Read the model definition and answer for the solid it produces. Units are mm, in the model's axes. Face numbers are marked on the shaded views. A direction names the side the tool comes from. Round coordinates to 2 decimals unless told otherwise and drop trailing zeros. Write each loop counter-clockwise with the first axis right and the second up, starting at its lowest first coordinate (ties: lowest second). Pieces come first, ordered by that corner, then holes. Notation, with made-up numbers: (59.25, 63) - (79.25, 63) arc R17 ccw to (79.25, 93) - close; hole circle Ø4 at (67.25, 75). An arc over 180 degrees is marked (long way). One line per item, written item: value. Start each with the question number.
(1) A cutting plane is placed at A-A, the plane z = 2. Determine the outline of the cut face in (x, y).
(2) A cutting plane is placed at B-B, the plane y = 41.75. Determine the outline of the cut face in (x, z), plus the area to 3 significant figures.
(3) Flat-ended cylindrical pins translate along their axes: pin 1 Ø4 at (y, z) = (43.5, 3) entering from +X; pin 2 Ø5 at (x, y) = (-19.5, 31) entering from -Z; pin 3 Ø2 at (x, z) = (48.5, 2) entering from +Y; pin 4 Ø5 at (y, z) = (-25, -37.41) entering from +X. Find the tip coordinate at first contact, or state that the pin passes through.
(4) A cutting plane is placed at C-C, the plane z = -37.41. Determine the outline of the cut face in (x, y) (3 decimals), plus the area to 3 significant figures.
(5) For the marked faces 1, 2 and 3, determine the directions among +Z, -Z, +X, -X, +Y, -Y from which every point of the face is accessible in a straight line to the end or side of a thin tool.
(6) Find the intervals of material crossed by L1, parallel to Y at x = 0, z = -37.41; L2, parallel to Y at x = 30.5, z = 2; L3, parallel to X at y = -32, z = -43.5 (3 decimals), in increasing order.
(7) A cutting plane is placed at D-D, the plane x = 29.5. Determine the outline of the cut face in (y, z).
from build123d import *

# Parameters (mm, degrees)
SKETCH1_W           = 100
SKETCH1_H           = 75
BOSS_EXTRUDE1_DEPTH = 4
SKETCH2_R           = 2
BOSS_EXTRUDE2_DEPTH = 30
SKETCH3_W           = 50
SKETCH3_H           = 25
BOSS_EXTRUDE3_DEPTH = 6.665
CUT_EXTRUDE2_START  = -13.33
CUT_EXTRUDE2_DEPTH  = 13.33
SKETCH5_R           = 4.2
CUT_EXTRUDE3_DEPTH  = 89.340164846


# Read off the part's stored shape, not the designer's step: Cut-Extrude2
with BuildPart() as part:
    # Sketch1 → Boss-Extrude1 (new body)
    with BuildSketch(Plane.XY):
        Rectangle(SKETCH1_W, SKETCH1_H)
    extrude(amount=BOSS_EXTRUDE1_DEPTH)

    # Sketch2 → Boss-Extrude2 (add)
    with BuildSketch(Plane(origin=(45, 0, 0), x_dir=(0, 0, -1), z_dir=(1, 0, 0))):
        with BuildLine():
            Line((-4, 38.285898385), (-4, 37.428468659))
            Line((-4, 37.428468659), (0, 37.428468659))
            Line((0, 37.428468659), (0, 38.285898385))
            ThreePointArc((0, 38.285898385), (-2, 45.75), (-4, 38.285898385))
        make_face()
        with Locations((-2, 41.75)):
            Circle(SKETCH2_R, mode=Mode.SUBTRACT)
    boss_extrude2 = extrude(amount=-BOSS_EXTRUDE2_DEPTH)

    # Mirror1: Boss-Extrude2 across plane
    add(boss_extrude2.mirror(Plane.ZY))

    # Sketch3 → Boss-Extrude3 (add, symmetric)
    with BuildSketch(Plane.ZY):
        with Locations((-25, -25)):
            Rectangle(SKETCH3_W, SKETCH3_H)
    extrude(amount=BOSS_EXTRUDE3_DEPTH, both=True)

    # Cut-Extrude2 outline → Cut-Extrude2 (cut)
    with BuildSketch(Plane.ZY.offset(6.665).offset(CUT_EXTRUDE2_START)):
        with BuildLine():
            Line((-50, -37.5), (-38.919370818, -37.5))
            ThreePointArc((-38.919370818, -37.5), (-46.831015832, -33.352603885), (-50, -25.000804036))
            Line((-50, -25.000804036), (-50, -37.5))
        make_face()
        with BuildLine():
            Line((-50, -12.5), (-50, -25.000804036))
            ThreePointArc((-50, -25.000804036), (-46.826545708, -16.643964506), (-38.905994132, -12.5))
            Line((-38.905994132, -12.5), (-50, -12.5))
        make_face()
    extrude(amount=CUT_EXTRUDE2_DEPTH, mode=Mode.SUBTRACT)

    # Sketch5 → Cut-Extrude3 (cut, through all)
    with BuildSketch(Plane.ZY.offset(6.665)):
        with Locations((-37.41, -25.000804036)):
            Circle(SKETCH5_R)
    extrude(amount=-CUT_EXTRUDE3_DEPTH, mode=Mode.SUBTRACT)


solid = part.part
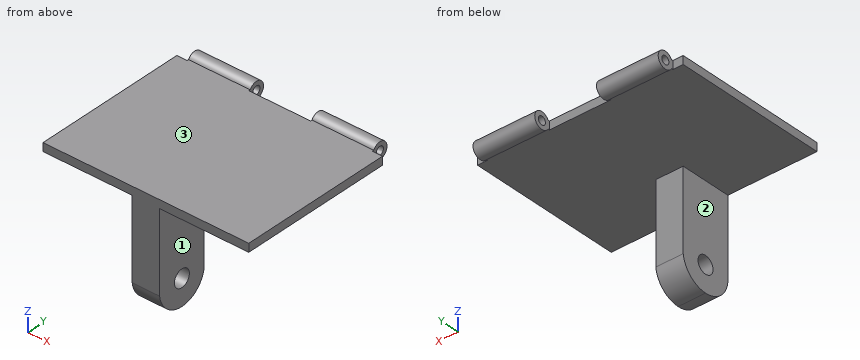
Here are the results:
1. outline: (-50, -37.5) - (50, -37.5) - (50, 37.5) - (45, 37.5) - (45, 39.75) - (15, 39.75) - (15, 37.5) - (-15, 37.5) - (-15, 39.75) - (-45, 39.75) - (-45, 37.5) - (-50, 37.5) - close; (-45, 43.75) - (-15, 43.75) - (-15, 45.75) - (-45, 45.75) - close; (15, 43.75) - (45, 43.75) - (45, 45.75) - (15, 45.75) - close
2. outline: (-45, -2) - (-15, -2) - (-15, 0) - (-45, 0) - close; (-45, 4) - (-15, 4) - (-15, 6) - (-45, 6) - close; (15, -2) - (45, -2) - (45, 0) - (15, 0) - close; (15, 4) - (45, 4) - (45, 6) - (15, 6) - close
2. area: 240 mm²
3. pin 1: x = 45
3. pin 2: z = 0
3. pin 3: y = 37.5
3. pin 4: through
4. outline: (-6.665, -37.5) - (6.665, -37.5) - (6.665, -29.201) - (-6.665, -29.201) - close; (-6.665, -20.801) - (6.665, -20.801) - (6.665, -12.5) - (-6.665, -12.5) - close
4. area: 221 mm²
5. face 1: -Z, +X, +Y, -Y
5. face 2: -Z, -X, +Y, -Y
5. face 3: +Z, +X, -X, -Y
6. L1: -37.5 to -29.2, -20.8 to -12.5
6. L2: -37.5 to 39.75, 43.75 to 45.75
6. L3: -6.665 to 6.665
7. outline: (-37.5, 0) - (38.29, 0) arc R4 ccw (long way) to (38.29, 4) - (-37.5, 4) - close; hole circle Ø4 at (41.75, 2)
